```python
from build123d import *

# Parameters (mm, degrees)
SKETCH_R        = 2.25
PAD_DEPTH       = 15
SKETCH001_R     = 7.6
POCKET_DEPTH    = 70.001
SKETCH002_R     = 4.6
POCKET001_DEPTH = 4
CHAMFER_SIZE    = 22


with BuildPart() as part:
    # Sketch → Pad (new body)
    with BuildSketch(Plane.XY):
        Polygon((-22.5, -35), (22.5, -35), (22.5, 5), (56.7, 5), (56.7, 25), (22.5, 25), (22.5, 35), (-22.5, 35), align=None)
        with Locations((-16.7, 30)):
            Circle(SKETCH_R, mode=Mode.SUBTRACT)
        with Locations((16.7, 30)):
            Circle(SKETCH_R, mode=Mode.SUBTRACT)
        with Locations((-16.7, -30)):
            Circle(SKETCH_R, mode=Mode.SUBTRACT)
        with Locations((16.7, -30)):
            Circle(SKETCH_R, mode=Mode.SUBTRACT)
        with Locations((-16.7, 0)):
            Circle(SKETCH_R, mode=Mode.SUBTRACT)
        with Locations((16.7, 0)):
            Circle(SKETCH_R, mode=Mode.SUBTRACT)
        with Locations((16.7, 15)):
            Circle(SKETCH_R, mode=Mode.SUBTRACT)
        with Locations((46.7, 15)):
            Circle(SKETCH_R, mode=Mode.SUBTRACT)
        with Locations((-16.7, 15)):
            Circle(SKETCH_R, mode=Mode.SUBTRACT)
        with Locations((28.3, 15)):
            Circle(SKETCH_R, mode=Mode.SUBTRACT)
    extrude(amount=PAD_DEPTH)

    # Sketch001 → Pocket (cut, through all)
    with BuildSketch(Plane.XZ.offset(35)):
        with Locations((0, 15)):
            Circle(SKETCH001_R)
    extrude(amount=-POCKET_DEPTH, mode=Mode.SUBTRACT)

    # Sketch002 → Pocket001 (cut)
    with BuildSketch(Plane.XY.offset(15)):
        with Locations((-16.7, 15)):
            Circle(SKETCH002_R)
        with Locations((16.7, 15)):
            Circle(SKETCH002_R)
        with Locations((28.3, 15)):
            Circle(SKETCH002_R)
        with Locations((46.7, 15)):
            Circle(SKETCH002_R)
    extrude(amount=-POCKET001_DEPTH, mode=Mode.SUBTRACT)

    # Chamfer
    chamfer_edges = [part.edges().sort_by_distance(p)[0] for p in [
        (22.5, 5, 7.5),
    ]]
    chamfer(chamfer_edges, length=CHAMFER_SIZE)


solid = part.part
```
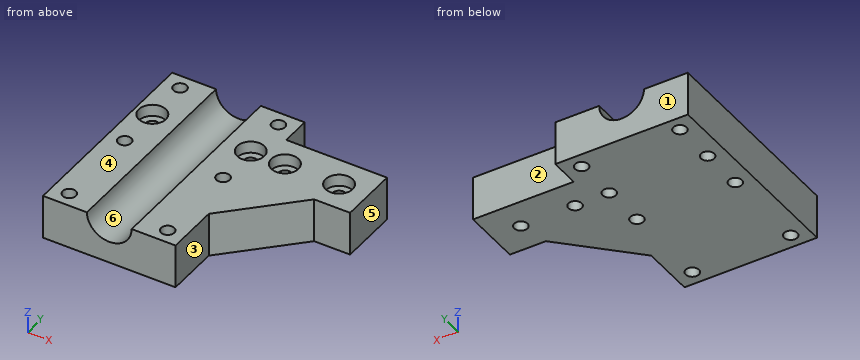
Input: part model. Units: mm. Frame: model coordinates. Face numbers are marked on the shaded views. A direction names the side the tool comes from. Give positions to 0.01 mm unless a question says otherwise; leave off trailing zeros. Loops run counter-clockwise (first coordinate to the right, second up) from the corner with the lowest first, then second, coordinate; pieces in that order, holes last. Notation, with made-up numbers: M -10,-16.75 L 29,-16.75 A32 ccw 29,14.25 Z; hole C 89.25,-34.75 d8. An arc over 180 degrees is marked long. Answer as CSV lines item,"result". Start each with the question number.
1. Section D-D on x = -16.7. Return loops of the section in (y, z).
2. Line query: L1, parallel to Y at x = 16.7, z = 2.5; L2, parallel to Y at x = 46.7, z = 6.5; L3, parallel to X at y = 29, z = 4.75. Output: solid intervals per line, ascending.
3. Reachability of the marked faces 1, 2 and 3 from +Z, -Z, +X, -X, +Y, -Y: full face, straight path, thin tool, end or side. Return the list, or none.
4. Section A-A on x = 28.3. Return loops of the section in (y, z), plus the area to 3 significant figures.
5. Pin query (flat end, axial travel): P1, Ø4.5, axis at y = -23, z = 7.5, coming from the +X side; P2, Ø3, axis at x = 39.5, z = 12.5, coming from the -Y side; P3, Ø7.5, axis at x = 35.5, z = 8.5, coming from the +Y side. Return the tip coordinate at first contact, or that it passes through.
6. Section B-B on z = 12.5. State how many separate pieces and enclosed holes the cut face has, plus the area to 3 significant figures.
7. Section C-C on y = 30. Return loops of the section in (x, z).
8. Pull-direction query (X, two-part tool) for the marked faces 4, 5 and 6; classes: released by +X, released by -X, zero draft, split by the parting line, or undercut.
Computed values:
1,outline,"M -35,0 L -32.25,0 L -32.25,15 L -35,15 Z; M -27.75,0 L -2.25,0 L -2.25,15 L -27.75,15 Z; M 2.25,0 L 12.75,0 L 12.75,11 L 10.4,11 L 10.4,15 L 2.25,15 Z; M 17.25,0 L 27.75,0 L 27.75,15 L 19.6,15 L 19.6,11 L 17.25,11 Z; M 32.25,0 L 35,0 L 35,15 L 32.25,15 Z"
2,L1,"y = -35 to -32.25, -27.75 to -2.25, 2.25 to 12.75, 17.25 to 27.75, 32.25 to 35"
2,L2,"y = 5 to 12.75, 17.25 to 25"
2,L3,"x = -22.5 to -18.72, -14.68 to 14.68, 18.72 to 22.5"
3,face 1,"+Z, -Z, +X, -X, +Y"
3,face 2,"+Z, -Z, +X, +Y"
3,face 3,"+Z, -Z, +X, -Y"
4,outline,"M -11.2,0 L 12.75,0 L 12.75,11 L 10.4,11 L 10.4,15 L -11.2,15 Z; M 17.25,0 L 25,0 L 25,15 L 19.6,15 L 19.6,11 L 17.25,11 Z"
4,area,"457 mm²"
5,P1,"stops at x = 22.5"
5,P2,"stops at y = -1.5"
5,P3,"stops at y = 25"
6,separate pieces,"2"
6,enclosed holes,"10"
6,area,"2,710 mm²"
7,outline,"M -22.5,0 L -18.95,0 L -18.95,15 L -22.5,15 Z; M -14.45,0 L 14.45,0 L 14.45,15 L 7.6,15 A7.6 cw -7.6,15 L -14.45,15 Z; M 18.95,0 L 22.5,0 L 22.5,15 L 18.95,15 Z"
8,face 4,"zero draft"
8,face 5,"released by +X"
8,face 6,"undercut"
